Input: part model. Units: mm. Frame: model coordinates. A direction names the side the tool comes from. Give positions to 0.01 mm unless a question says otherwise; leave off trailing zeros. Order: outer loops, then holes, each group sorted by start corner. A loop starts at its lowest first (then second) coordinate and runs counter-clockwise, first axis right, second up. Notation, with made-up numbers: (-12.5, 47.5) - (4.5, 47.5) arc R21 cw to (4.5, 58.5) - close; hole circle Ø2 at (3.5, -37). An arc over 180 degrees is marked (long way). Answer in a Markdown table with one row per item. Add a question column.
from build123d import *

# Parameters (mm, degrees)
SKETCH1_R           = 19.75
SKETCH1_R_2         = 6.985
SKETCH1_R_3         = 1.75
BOSS_EXTRUDE1_DEPTH = 6.35
CUT_EXTRUDE1_DEPTH  = 7.35
CIRPATTERN1_COUNT   = 3
CIRPATTERN1_ANGLE   = 60


with BuildPart() as part:
    # Sketch1 → Boss-Extrude1 (new body)
    with BuildSketch(Plane(origin=(0, 0, 0), x_dir=(1, 0, 0), z_dir=(0, 1, 0))):
        Circle(SKETCH1_R)
        Circle(SKETCH1_R_2, mode=Mode.SUBTRACT)
        with Locations((-14.289419162, 8.25)):
            Circle(SKETCH1_R_3, mode=Mode.SUBTRACT)
        with Locations((0, -16.5)):
            Circle(SKETCH1_R_3, mode=Mode.SUBTRACT)
        with Locations((14.289419162, 8.25)):
            Circle(SKETCH1_R_3, mode=Mode.SUBTRACT)
    extrude(amount=BOSS_EXTRUDE1_DEPTH)

    # Sketch2 → Cut-Extrude1 (cut, through all)
    with BuildSketch(Plane(origin=(0, 6.35, 0), x_dir=(1, 0, 0), z_dir=(0, 1, 0))):
        with BuildLine():
            ThreePointArc((8.036161973, 16.182379357), (7.2975, 12.639640768), (9.99627063, 15.050710096))
            ThreePointArc((9.99627063, 15.050710096), (10.255103275, 16.120005739), (11.354562521, 16.159715652))
            ThreePointArc((11.354562521, 16.159715652), (9.875, 17.104001725), (8.317443012, 17.913197418))
            ThreePointArc((8.317443012, 17.913197418), (8.832782842, 16.941182824), (8.036161973, 16.182379357))
        make_face()
    cut_extrude1 = extrude(amount=-CUT_EXTRUDE1_DEPTH, mode=Mode.SUBTRACT)

    # CirPattern1: Cut-Extrude1 ×3 about axis
    cirpattern1_axis = Axis((0, 0, 0), (0, 1, 0))
    for i in range(1, CIRPATTERN1_COUNT):
        add(cut_extrude1.rotate(cirpattern1_axis, i * CIRPATTERN1_ANGLE / (CIRPATTERN1_COUNT - 1)), mode=Mode.SUBTRACT)


solid = part.part
Q1. Section D-D, the plane z = -13. Return loops of the section in (x, y).
Q2. Pull-direction query (X, two-part tool) for faces 3 (the cylindrical face through (-5.07, 3.13, -19.09)), 4 (the cylindrical face through (-0.909, 3.131, -6.926)), 5 (the cylindrical face through (7.2, 3.2, -12.7)), 6 (the cylindrical face through (-0.699, 3.131, 19.738)); classes: +X half, -X half, draft (parallel to the pull), parting line (faces both ways), or undercut.
Q3. Section A-A, the plane z = 0. Return loops of the section in (x, y) (3 decimals).
Q4. Section B-B, the plane x = 0. Return loops of the section in (y, z) (3 decimals), then the cut area to 3 significant figures.
Q5. Contact query for flat-ended pins moving along their axis: P1, Ø2, axis at x = 5.5, y = 2, coming from the +Z side; P2, Ø3, axis at y = 4, z = -11, coming from the +X side; P3, Ø1.5, axis at y = 5.5, z = -14, coming from the -X side. Output: stop coordinate, or through.
Q6. Access query for faces 1 (the flat face through (0, 0, 9)), 2 (the cylindrical face through (-8.83, 3.22, -16.92)). Directions: +Z, -Z, +X, -X, +Y, -Y. A direction counts if a zero-diameter tool reaches every point of the face in a straight line with its end or side. Return the directions, or none.
Q7. Line query: probe 1 along Z at (x, y) = (0, 1.5) (3 decimals); probe 2 along X at (y, z) = (2.75, 16.5); probe 3 along X at (y, z) = (2.25, -2.5). Output: solid intervals per line, ascending.
Q8. Section C-C, the plane y = 1. Return loops of the section in (x, z) (3 decimals).
Computed:
| question | item | result |
|---|---|---|
| 1 | outline | (-14.87, 0) - (-9.65, 0) - (-9.65, 6.35) - (-14.87, 6.35) - close; (-6.85, 0) - (6.85, 0) - (6.85, 6.35) - (-6.85, 6.35) - close; (9.65, 0) - (14.87, 0) - (14.87, 6.35) - (9.65, 6.35) - close |
| 2 | face 3 | -X half |
| 2 | face 4 | undercut |
| 2 | face 5 | undercut |
| 2 | face 6 | parting line |
| 3 | outline | (-19.75, 0) - (-6.985, 0) - (-6.985, 6.35) - (-19.75, 6.35) - close; (6.985, 0) - (19.75, 0) - (19.75, 6.35) - (6.985, 6.35) - close |
| 4 | outline | (0, -14.595) - (6.35, -14.595) - (6.35, -6.985) - (0, -6.985) - close; (0, 6.985) - (6.35, 6.985) - (6.35, 14.75) - (0, 14.75) - close; (0, 18.25) - (6.35, 18.25) - (6.35, 19.75) - (0, 19.75) - close |
| 4 | area | 107 mm^2 |
| 5 | P1 | stops at z = 19.23 |
| 5 | P2 | stops at x = 17.32 |
| 5 | P3 | stops at x = -14.65 |
| 6 | face 1 | +Z, -Z, +X, -X, -Y |
| 6 | face 2 | +Y, -Y |
| 7 | probe 1 | z = -14.595 to -6.985, 6.985 to 14.75, 18.25 to 19.75 |
| 7 | probe 2 | x = -10.85 to -1.75, 1.75 to 10.85 |
| 7 | probe 3 | x = -19.59 to -6.52, 6.52 to 19.59 |
| 8 | outline | (-11.355, -16.16) arc R0.911 ccw to (-9.996, -15.051) arc R1.905 cw (long way) to (-8.036, -16.182) arc R0.911 ccw to (-8.317, -17.913) arc R19.75 ccw to (-1.753, -19.672) arc R0.911 ccw to (-1.132, -18.032) arc R1.905 cw (long way) to (1.132, -18.032) arc R0.911 ccw to (1.753, -19.672) arc R19.75 ccw to (8.317, -17.913) arc R0.911 ccw to (8.036, -16.182) arc R1.905 cw (long way) to (9.996, -15.051) arc R0.911 ccw to (11.355, -16.16) arc R19.75 ccw (long way) to start; hole circle Ø3.5 at (-14.289, -8.25); hole circle Ø13.97 at (0, 0); hole circle Ø3.5 at (0, 16.5); hole circle Ø3.5 at (14.289, -8.25) |
